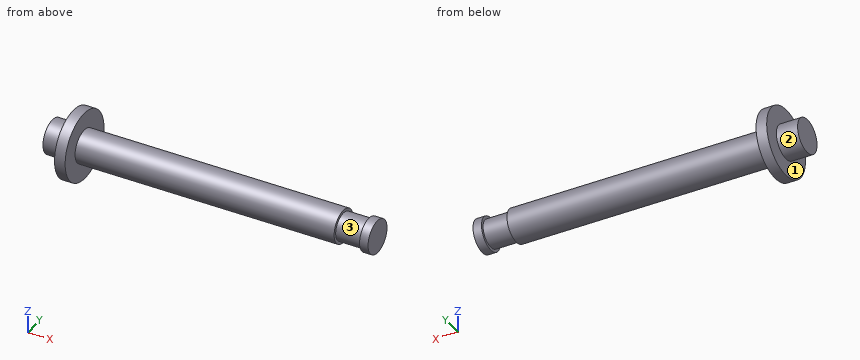
Autodesk Inventor part; units mm, degrees
ref_plane "YZ Plane" through (0, 0, 0) normal (1, 0, 0) x (0, 1, 0)
ref_plane "XZ Plane" through (0, 0, 0) normal (0, 1, 0) x (-1, 0, 0)
ref_plane "XY Plane" through (0, 0, 0) normal (0, 0, 1) x (1, 0, 0)
sketch "Sketch1" plane through (0, 0, 0) normal (0, 0, 1) x (1, 0, 0)
  line L0 (0, 0) -> (2.5, 0)
  line L1 (2.5, 0) -> (2.5, 2)
  line L2 (2.5, 2) -> (0, 2)
  line L3 (0, 2) -> (0, 0)
  line L4 (2.5, 0) -> (3.75, 0)
  line L5 (3.75, 0) -> (3.75, 4)
  line L6 (3.75, 4) -> (2.5, 4)
  line L7 (2.5, 4) -> (2.5, 0)
  line L8 (3.75, 0) -> (34.25, 0)
  line L9 (34.25, 0) -> (34.25, 1.95)
  line L10 (34.25, 1.95) -> (3.75, 1.95)
  line L11 (3.75, 1.95) -> (3.75, 0)
  line L12 (34.25, 0) -> (37.25, 0)
  line L13 (37.25, 0) -> (37.25, 1.625)
  line L14 (37.25, 1.625) -> (34.25, 1.625)
  line L15 (34.25, 1.625) -> (34.25, 0)
  line L16 (37.25, 0) -> (38.25, 0)
  line L17 (38.25, 0) -> (38.25, 1.95)
  line L18 (38.25, 1.95) -> (37.25, 1.95)
  line L19 (37.25, 1.95) -> (37.25, 0)
  dimension "d0" = 4
  dimension "d1" = 8
  dimension "d2" = 3.9
  dimension "d3" = 3.25
  dimension "d4" = 2.5
  dimension "d5" = 3.75
  dimension "d6" = 34.25
  dimension "d7" = 37.25
  dimension "d8" = 38.25
revolve "Revolution1" add sketch "Sketch1" angle 360 about axis through (3.75, 0, 0) along (1, 0, 0)
properties part number "403-06" material "Steel, Mild"
Work out the finished part from the listing and answer in its coordinate system (mm). Face numbers are marked on the shaded views. Round coordinates to 2 decimals unless told otherwise and drop trailing zeros. Order: outer loops, then holes, each group sorted by start corner. A loop starts at its lowest first (then second) coordinate and runs counter-clockwise, first axis right, second up.
Q1. A cutting plane is placed at A-A, the plane z = 0. Determine the outline of the cut face in (x, y) (3 decimals).
Solution:
outline: (0, -2) - (2.5, -2) - (2.5, -4) - (3.75, -4) - (3.75, -1.95) - (34.25, -1.95) - (34.25, -1.625) - (37.25, -1.625) - (37.25, -1.95) - (38.25, -1.95) - (38.25, 1.95) - (37.25, 1.95) - (37.25, 1.625) - (34.25, 1.625) - (34.25, 1.95) - (3.75, 1.95) - (3.75, 4) - (2.5, 4) - (2.5, 2) - (0, 2) - close
Q2. The mould has two halves that part along X. Classify the marked faces 1, 2 and 3: pulls with the +X half, pulls with the -X half, needs draft (parallel to the pull), parting line crosses it, or undercut.
Solution:
face 1: pulls with the -X half
face 2: needs draft
face 3: undercut
Q3. Find the intervals of material crossed by line 1 along X through (y, z) = (-3, 1.5); line 2 along Z through (x, y) = (35.5, -1); line 3 along Y through (x, z) = (24, 1.5), in increasing order.
Solution:
line 1: x = 2.5 to 3.75
line 2: z = -1.28 to 1.28
line 3: y = -1.25 to 1.25
Q4. Given pin 1 Ø1 at (x, y) = (21, 2) entering from +Z; pin 2 Ø2 at (x, z) = (21.5, -0.5) entering from -Y; pin 3 Ø4 at (x, y) = (29, 1) entering from +Z, each flat-ended and moving along its own axis, determine where each tip first touches the part or whether it passes through.
Solution:
pin 1: stops at z = 1.25
pin 2: stops at y = -1.95
pin 3: stops at z = 1.95
Q5. A cutting plane is placed at D-D, the plane x = 23. Determine the outline of the cut face in (y, z), then the cut area to 3 significant figures.
Solution:
outline: circle Ø3.9 at (0, 0)
area: 11.9 mm2
Q6. A cutting plane is placed at C-C, the plane x = 35. Determine the outline of the cut face in (y, z) (3 decimals), then the cut area to 3 significant figures.
Solution:
outline: circle Ø3.25 at (0, 0)
area: 8.30 mm2
